Design review of the part shown in the three views and the two pictorial views. Dimensions are in mm from the part's minimum x, y and z. A direction names the side the tool comes from. Coordinates: 2 decimals unless noted, no trailing zeros. Write each loop counter-clockwise with the first axis right and the second up, starting at its lowest first coordinate (ties: lowest second). Pieces come first, ordered by that corner, then holes.
Q1. For L1, parallel to Y at x = 6.25, z = 10; L2, parallel to Z at x = 7, y = 22.5; L3, parallel to Z at x = 4.5, y = 22.5, list the stretches that pass through material, from the lowest coordinate up.
Q2. For pin 1 Ø5 at (x, z) = (5, 28) entering from -Y; pin 2 Ø1.5 at (x, y) = (6, 15.5) entering from +Z, all flat-tipped, find the tip position at first contact; note any pin that passes through.
Q3. Take a section at C-C, the plane z = 10. Write out the cut boundary in (x, y).
Q4. Take a section at B-B, the plane x = 2. Write out the cut boundary in (y, z), plus the area to 3 significant figures.
Q5. Take a section at D-D, the plane y = 16.5. Write out the cut boundary in (x, z), plus the area to 3 significant figures.
Q6. For the marked faces 1 and 2, list the 3-axis set-ups (+Z, -Z, +X, -X, +Y, -Y) from which the entire face can be reached by the end or side of a thin tool; tool diameter is ignored.
Q7. The part is to be moulded in two halves that separate along X. For the marked faces 3, 4 and 5, say which applies: released by +X, released by -X, zero draft, split by the parting line, or undercut.
Q8. Take a section at A-A, the plane y = 22.5. Write out the cut boundary in (x, z), plus the area to 3 significant figures.
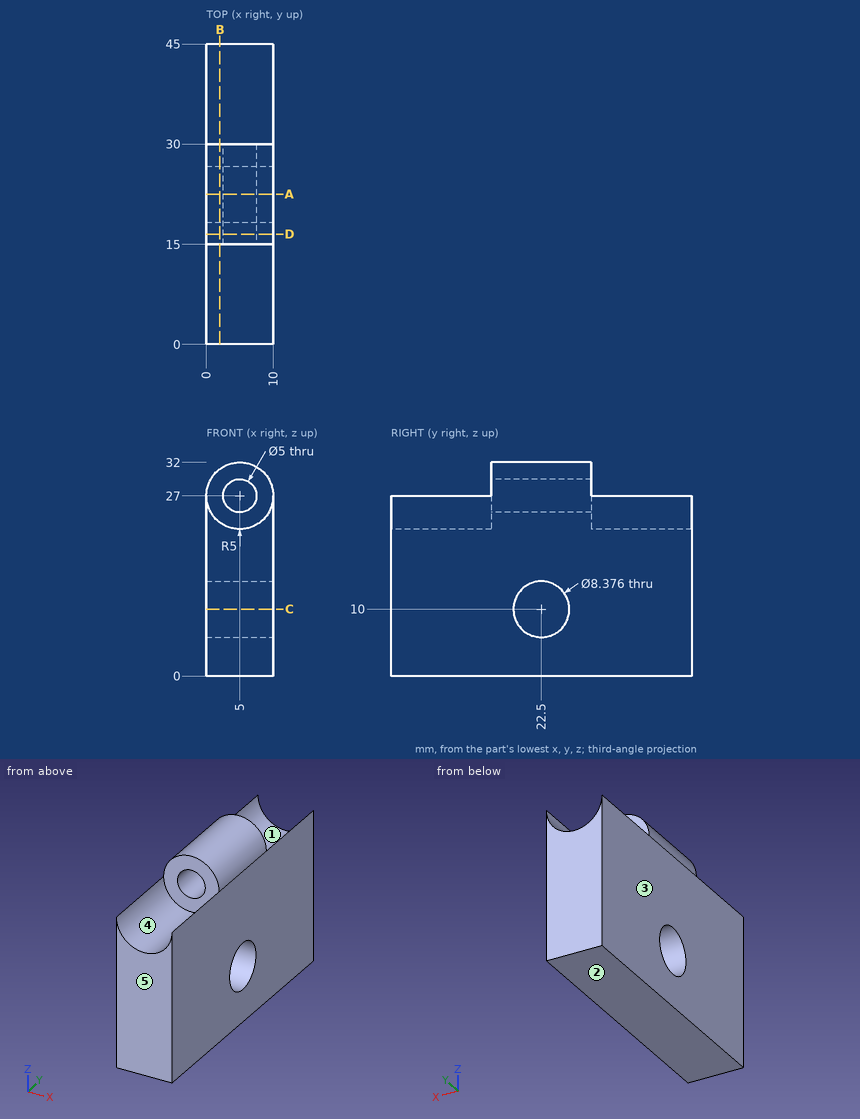
Responses:
1. L1: y = 0 to 18.31, 26.69 to 45
1. L2: z = 0 to 5.81, 14.19 to 25.5, 28.5 to 31.58
1. L3: z = 0 to 5.81, 14.19 to 24.55, 29.45 to 31.97
2. pin 1: stops at y = 15
2. pin 2: stops at z = 31.99
3. outline: (0, 0) - (10, 0) - (10, 18.31) - (0, 18.31) - close; (0, 26.69) - (10, 26.69) - (10, 45) - (0, 45) - close
4. outline: (0, 0) - (45, 0) - (45, 23) - (30, 23) - (30, 31) - (15, 31) - (15, 23) - (0, 23) - close; hole circle Ø8.38 at (22.5, 10)
4. area: 1,100 mm2
5. outline: (0, 0) - (10, 0) - (10, 27) arc R5 ccw to (0, 27) - close; hole circle Ø5 at (5, 27)
5. area: 290 mm2
6. face 1: +Z, +Y
6. face 2: -Z, +X, -X, +Y, -Y
7. face 3: released by -X
7. face 4: undercut
7. face 5: zero draft
8. outline: (0, 0) - (10, 0) - (10, 5.81) - (0, 5.81) - close; (0, 14.19) - (10, 14.19) - (10, 27) arc R5 ccw to (0, 27) - close; hole circle Ø5 at (5, 27)
8. area: 206 mm2
